from build123d import *

# Parameters (mm, degrees)
BOSS_EXTRUDE1_DEPTH     = 2
CUT_EXTRUDE2_DEPTH      = 98.534609242
CUT_EXTRUDE2_DEPTH_BACK = 98.534609242
CIRPATTERN2_START       = -2
CIRPATTERN2_DEPTH       = 4


# Read off the part's stored shape, not the designer's step: CirPattern2
with BuildPart() as part:
    # Sketch1 → Boss-Extrude1 (new, symmetric)
    with BuildSketch(Plane(origin=(0, 0, 0), x_dir=(1, 0, 0), z_dir=(0, 1, 0))):
        with BuildLine():
            Line((25, 5), (97, 5))
            Line((97, 5), (97, -5))
            Line((97, -5), (25, -5))
            ThreePointArc((25, -5), (17.09430585, -6.282917549), (10, -10))
            Line((10, -10), (0, -10))
            Line((0, -10), (0, 10))
            Line((0, 10), (10, 10))
            ThreePointArc((10, 10), (17.09430585, 6.282917549), (25, 5))
        make_face()
    extrude(amount=BOSS_EXTRUDE1_DEPTH, both=True)

    # Sketch2<3> → Cut-Extrude2 (cut, two sides: drawn at the far end of the back side and taken through both)
    with BuildSketch(Plane(origin=(0, 0, 0), x_dir=(1, 0, 0), z_dir=(0, 1, 0)).offset(-CUT_EXTRUDE2_DEPTH_BACK)):
        Polygon((75, 5), (75, 0), (80.958767963, -5), (97, -5), (97, 5), align=None)
        Polygon((80.958767963, -5), (75, 0), (75, -5), align=None)
    extrude(amount=CUT_EXTRUDE2_DEPTH + CUT_EXTRUDE2_DEPTH_BACK, mode=Mode.SUBTRACT)

    # CirPattern2 outline → CirPattern2 (add)
    with BuildSketch(Plane(origin=(0, 0, 0), x_dir=(1, 0, 0), z_dir=(0, 1, 0)).offset(CIRPATTERN2_START)):
        with BuildLine():
            Line((0, 10), (-10, 10))
            ThreePointArc((-10, 10), (-17.09430585, 6.282917549), (-25, 5))
            Line((-25, 5), (-75, 5))
            Line((-75, 5), (-75, -5))
            Line((-75, -5), (-25, -5))
            ThreePointArc((-25, -5), (-17.09430585, -6.282917549), (-10, -10))
            Line((-10, -10), (0, -10))
            Line((0, -10), (0, 10))
        make_face()
    extrude(amount=CIRPATTERN2_DEPTH)


solid = part.part
Work out the finished part from the listing and answer in its coordinate system (mm). A direction names the side the tool comes from. Round coordinates to 2 decimals unless told otherwise and drop trailing zeros. Loops run counter-clockwise (first coordinate to the right, second up) from the corner with the lowest first, then second, coordinate; pieces in that order, holes last. Notation, with made-up numbers: M 73,36.25 L 113,36.25 A33 cw 113,73.25 Z; hole C 78.5,54.25 d5. An arc over 180 degrees is marked long. One line per question, with ' | ' between items. Start each with the question number.
(1) A cutting plane is placed at A-A on y = 0.2. Write down the section's boundary in (x, z), plus the area to 3 significant figures.
(2) A cutting plane is placed at C-C on z = -7.75. Write down the section's boundary in (x, y), plus the area to 3 significant figures.
(3) Find the intervals of material crossed by line 1 (Z direction, x = 57, y = 0.55); line 2 (Z direction, x = -16, y = 1.7); line 3 (X direction, y = 0.3, z = 7.75), in increasing order.
(4) Flat-ended cylindrical pins translate along their axes: pin 1 Ø1.2 at (x, y) = (-61.5, -0.5) entering from -Z; pin 2 Ø1.2 at (x, y) = (-54, -1) entering from +Z; pin 3 Ø2 at (x, y) = (20.5, 1.5) entering from +Z. Find the tip coordinate at first contact, or state that the pin passes through.
(5) A tool of negligible diameter and unlimited length cuts with its end or side. For faces 1 (the face through (50, 0, -5)), 2 (the face through (50, 0, 5)), 3 (the face through (-50, 0, 5)), 4 (the face through (-50, 0, -5)), from which of +Z, -Z, +X, -X, +Y, -Y can it reach the whole face along a straight path? Write none if from no direction.
(6) A cutting plane is placed at B-B on x = -47.5. Write down the section's boundary in (y, z).
Geometry check:
1) outline: M -75,-5 L -25,-5 A25 cw -10,-10 L 10,-10 A25 cw 25,-5 L 75,-5 L 75,5 L 25,5 A25 cw 10,10 L -10,10 A25 cw -25,5 L -75,5 Z | area: 1,800 mm²
2) outline: M -13.6,-2 L 13.6,-2 L 13.6,2 L -13.6,2 Z | area: 109 mm²
3) line 1: z = -5 to 5 | line 2: z = -6.68 to 6.68 | line 3: x = -13.6 to 13.6
4) pin 1: stops at z = -5 | pin 2: stops at z = 5 | pin 3: stops at z = 5.61
5) face 1: -Z, +X, +Y, -Y | face 2: +Z, +X, +Y, -Y | face 3: +Z, -X, +Y, -Y | face 4: -Z, -X, +Y, -Y
6) outline: M -2,-5 L 2,-5 L 2,5 L -2,5 Z
